Here's how the part is built. I have some questions about the finished solid (model axes, mm). A direction names the side the tool comes from. Coordinates: 2 decimals unless noted, no trailing zeros. Order: outer loops, then holes, each group sorted by start corner. A loop starts at its lowest first (then second) coordinate and runs counter-clockwise, first axis right, second up. Notation, with made-up numbers: (21.25, 15.5) - (77.25, 15.5) arc R32 cw to (77.25, 53.5) - close; hole circle Ø7 at (50, 10.25). An arc over 180 degrees is marked (long way). Use CSV: the item, a comma, the result in double quotes. Start each with the question number.
from build123d import *

# Parameters (mm, degrees)
BOSS_EXTRUDE2_DEPTH = 20
BOSS_EXTRUDE3_DEPTH = 20


with BuildPart() as part:
    # Sketch1 → Boss-Extrude2 (new body)
    with BuildSketch(Plane.XY):
        Polygon((-2.274774775, 3.513513514), (-14.774774775, 3.513513514), (-14.774774775, 15.540540541), (5.225225225, 15.540540541), (15.225225225, 15.540540541), (15.225225225, -9.459459459), (5.225225225, -9.459459459), (5.225225225, 8.513513514), (-2.274774775, 8.513513514), align=None)
    extrude(amount=BOSS_EXTRUDE2_DEPTH)

    # Sketch2 → Boss-Extrude3 (add)
    with BuildSketch(Plane.XY.offset(20)):
        Polygon((-14.774774775, 15.540540541), (20.580564285, 50.8958796), (22.701884628, 48.774559256), (2.346545569, 28.419220197), (15.225225225, 15.540540541), (12.3967981, 15.540540541), (0.932332006, 27.005006635), (-10.532134088, 15.540540541), align=None)
    extrude(amount=-BOSS_EXTRUDE3_DEPTH)


solid = part.part
Item 1: Please list where these lines run through material, in increasing order: line 1 along Y through (x, z) = (3, 14.75); line 2 along Y through (x, z) = (12, 6.25); line 3 along X through (y, z) = (5, 16). Write a range as from..to.
Item 2: We'd pull the mould along Y, two halves only. Please class faces 1 (the flat face through (2.655, 32.971, 10.14)), 2 (the flat face through (6.745, 21.193, 10.14)), 3 (the flat face through (10, -9.459, 10)): released by +Y, released by -Y, zero draft, split by the parting line, or undercut.
Item 3: For pin 1 Ø1.5 at (x, z) = (-9.5, 16.5) entering from +Y; pin 2 Ø12 at (y, z) = (42, 6.5) entering from -X; pin 3 Ø6 at (x, z) = (-8.5, 9.5) entering from -Y, each with a flat end and sliding along its axis, tell me the tip position at first contact or that it passes through.
Item 4: For faces 4 (the flat face through (8.696, 22.07, 10.14)), 5 (the flat face through (5.225, -1, 10)), 6 (the flat face through (1, 15.541, 10)), which set-ups out of +Z, -Z, +X, -X, +Y, -Y let a thin tool reach every point of the face, with its end or its side?
Item 5: Suppose I cut it at D-D on x = 9. Write out the boundary of the cut face in (y, z).
Item 6: Suppose I cut it at A-A on z = 3. Write out the boundary of the cut face in (x, y) (3 decimals).
Item 7: Suppose I cut it at B-B on y = 23.5. Write out the boundary of the cut face in (x, z), then the cut area to 3 significant figures.
Item 8: Suppose I cut it at C-C on x = -9.5. Write out the boundary of the cut face in (y, z).
Here are the results:
1,line 1,"8.51..15.54, 24.94..27.77, 29.07..33.32"
1,line 2,"-9.46..15.54, 15.94..18.77, 38.07..42.32"
1,line 3,"-14.77..-2.27, 5.23..15.23"
2,face 1,"released by +Y"
2,face 2,"undercut"
2,face 3,"released by -Y"
3,pin 1,"y = 21.57"
3,pin 2,"x = 5.68"
3,pin 3,"y = 3.51"
4,face 4,"+Z, -Z, +X"
4,face 5,"+Z, -Z, -Y"
4,face 6,"+Z, -Z"
5,outline,"(-9.46, 0) - (15.54, 0) - (15.54, 20) - (-9.46, 20) - close; (18.94, 0) - (21.77, 0) - (21.77, 20) - (18.94, 20) - close; (35.07, 0) - (39.32, 0) - (39.32, 20) - (35.07, 20) - close"
6,outline,"(-14.775, 3.514) - (-2.275, 3.514) - (-2.275, 8.514) - (5.225, 8.514) - (5.225, -9.459) - (15.225, -9.459) - (15.225, 15.541) - (2.347, 28.419) - (22.702, 48.775) - (20.581, 50.896) - (-14.775, 15.541) - close; hole (-10.532, 15.541) - (12.397, 15.541) - (0.932, 27.005) - close"
7,outline,"(-6.82, 0) - (-2.57, 0) - (-2.57, 20) - (-6.82, 20) - close; (4.44, 0) - (7.27, 0) - (7.27, 20) - (4.44, 20) - close"
7,area,"141 mm^2"
8,outline,"(3.51, 0) - (15.54, 0) - (15.54, 20) - (3.51, 20) - close; (16.57, 0) - (20.82, 0) - (20.82, 20) - (16.57, 20) - close"
